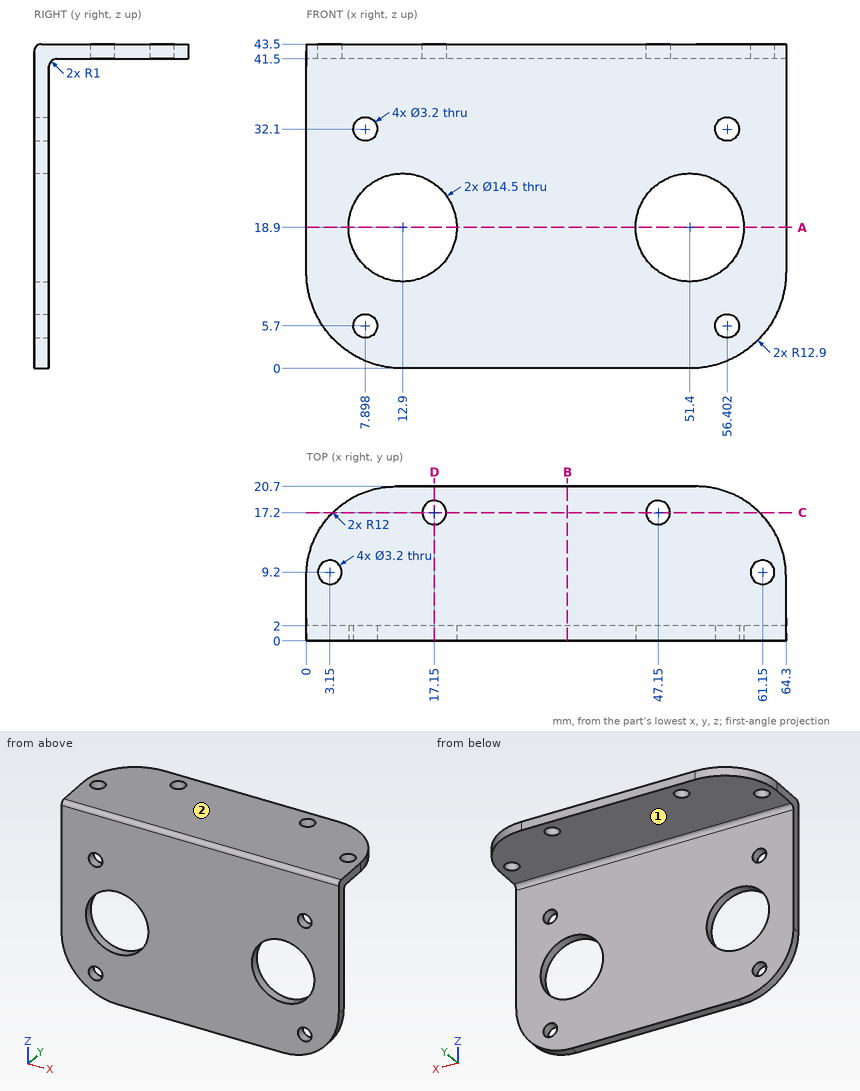
Study the drawing (mm; zero at the part's minimum x, y, z) and answer. A direction names the side the tool comes from. Give positions to 0.01 mm unless a question says otherwise; leave off trailing zeros. Order: outer loops, then holes, each group sorted by start corner. A loop starts at its lowest first (then second) coordinate and runs counter-clockwise, first axis right, second up.
1) Find section A-A on z = 18.9. Write down the section's boundary in (x, y).
Reported:
outline: (0, 0) - (5.65, 0) - (5.65, 2) - (0, 2) - close; (20.15, 0) - (44.15, 0) - (44.15, 2) - (20.15, 2) - close; (58.65, 0) - (64.3, 0) - (64.3, 2) - (58.65, 2) - close
2) Consider line 1 along X through (y, z) = (1.15, 32.1); line 2 along Z through (x, y) = (60, 7); line 3 along Y through (x, z) = (18.5, 38). Determine where each line is inside the solid, lowest interval first.
Reported:
line 1: x = 0 to 6.3, 9.5 to 54.8, 58 to 64.3
line 2: z = 41.5 to 43.5
line 3: y = 0 to 2
3) Find section C-C on y = 17.2. Write down the section's boundary in (x, z), then the cut area to 3 significant figures.
Reported:
outline: (3.53, 41.5) - (15.55, 41.5) - (15.55, 43.5) - (3.53, 43.5) - close; (18.75, 41.5) - (45.55, 41.5) - (45.55, 43.5) - (18.75, 43.5) - close; (48.75, 41.5) - (60.77, 41.5) - (60.77, 43.5) - (48.75, 43.5) - close
area: 102 mm2
4) Find section B-B on x = 35. Write down the section's boundary in (y, z).
Reported:
outline: (0, 0) - (2, 0) - (2, 40.5) arc R1 cw to (3, 41.5) - (20.7, 41.5) - (20.7, 43.5) - (1, 43.5) arc R1 ccw to (0, 42.5) - close
5) Given P1, Ø1.9, axis at x = 47.15, y = 17.2, coming from the -Z side; P2, Ø3.5, axis at x = 56.4, z = 5.7, coming from the -Y side; P3, Ø4, axis at x = 41.5, z = 33.5, coming from the +Y side; P4, Ø10, axis at x = 33, y = 17.5, coming from the -Z side, each flat-ended and moving along its own axis, determine where each tip first touches the part or whether it passes through.
Reported:
P1: passes through
P2: stops at y = 0
P3: stops at y = 2
P4: stops at z = 41.5
6) For the marked faces 1 and 2, determine the directions among +Z, -Z, +X, -X, +Y, -Y from which every point of the face is accessible in a straight line to the end or side of a thin tool.
Reported:
face 1: -Z, +X, -X, +Y
face 2: +Z, +X, -X, +Y, -Y
7) Find section D-D on x = 17.15. Write down the section's boundary in (y, z).
Reported:
outline: (0, 0) - (2, 0) - (2, 13.03) - (0, 13.03) - close; (0, 24.77) - (2, 24.77) - (2, 40.5) arc R1 cw to (3, 41.5) - (15.6, 41.5) - (15.6, 43.5) - (1, 43.5) arc R1 ccw to (0, 42.5) - close; (18.8, 41.5) - (20.7, 41.5) - (20.7, 43.5) - (18.8, 43.5) - close
